Input: part model. Units: mm. Frame: model coordinates. A direction names the side the tool comes from. Round coordinates to 2 decimals unless told otherwise and drop trailing zeros. Order: outer loops, then holes, each group sorted by start corner. A loop starts at its lowest first (then second) coordinate and runs counter-clockwise, first axis right, second up. Notation, with made-up numbers: (-30.75, -11.5) -> (13.25, -11.5) arc R16 ccw to (13.25, 5.5) -> close; hole circle Ø6 at (89.5, 74.5). An arc over 180 degrees is marked (long way). Use a Markdown table: item, result.
Autodesk Inventor part; units mm, degrees
ref_plane "YZ Plane" through (0, 0, 0) normal (1, 0, 0) x (0, 1, 0)
ref_plane "XZ Plane" through (0, 0, 0) normal (0, 1, 0) x (-1, 0, 0)
ref_plane "XY Plane" through (0, 0, 0) normal (0, 0, 1) x (1, 0, 0)
sketch "Sketch1" plane through (0, 0, 0) normal (0, 1, 0) x (-1, 0, 0)
  circle A0 centre (0, 0) radius 1.5
  circle A1 centre (0, 0) radius 5.5
  circle A2 centre (0, -18) radius 5
  line L0 (5.4979, -0.1528) -> (4.9981, -18.1389)
  line L1 (-4.9981, -18.1389) -> (-5.4979, -0.1528)
  line L2 (0, 0) -> (0, 15) construction
  line L3 (-3.4, 0) -> (-3.4, 15)
  line L4 (3.4, 15) -> (3.4, 0)
  arc A3 (-3.4, 0) -> (3.4, 0) centre (0, 0) ccw
  arc A4 (3.4, 15) -> (-3.4, 15) centre (0, 15) ccw
  arc A5 (3.4, 7.5) -> (4.7003, 2.8561) centre (12.3429, 7.5) ccw
  arc A6 (-4.7003, 2.8561) -> (-3.4, 7.5) centre (-12.3429, 7.5) ccw
  point P0 (0, 7.5)
  point P1 (-3.4, 4.3232)
  point P2 (3.4, 4.3232)
  point P3 (-3.4, 7.5)
  dimension "d0" = 3
  dimension "d1" = 11
  dimension "d3" = 18
  dimension "d43" = 15
  dimension "d44" = 3.4
  dimension "d74" = 10
extrude "Extrusion1" add sketch "Sketch1" along normal blind 4
sketch "Sketch2" plane through (0, 4, 0) normal (0, 1, 0) x (1, 0, 0)
  arc A0 (4.9981, 18.1389) -> (-4.9981, 18.1389) centre (0, 18) ccw
  circle A1 centre (0, 0) radius 1.5
  line L0 (0, 16.8) -> (0, 12) construction
  line L1 (-2.6, 16.8) -> (-2.6, 12)
  line L2 (2.6, 12) -> (2.6, 16.8)
  arc A2 (2.6, 16.8) -> (-2.6, 16.8) centre (0, 16.8) ccw
  arc A3 (-2.6, 12) -> (2.6, 12) centre (0, 12) ccw
  line L3 (-3.4, -7.5) -> (-3.4, -15)
  arc A4 (-3.4, -15) -> (3.4, -15) centre (0, -15) ccw
  line L4 (3.4, -15) -> (3.4, -7.5)
  line L5 (-4.9981, 18.1389) -> (-5.4979, 0.1528)
  arc A5 (-5.4979, 0.1528) -> (-4.7003, -2.8561) centre (0, 0) ccw
  arc A6 (4.7003, -2.8561) -> (5.4979, 0.1528) centre (0, 0) ccw
  line L6 (5.4979, 0.1528) -> (4.9981, 18.1389)
  arc A7 (-3.4, -7.5) -> (-4.7003, -2.8561) centre (-12.3429, -7.5) ccw
  arc A8 (4.7003, -2.8561) -> (3.4, -7.5) centre (12.3429, -7.5) ccw
  point P0 (0, 14.4)
  dimension "d6" = 4.8
  dimension "d7" = 5.2
  dimension "d9" = 12
extrude "Extrusion2" cut sketch "Sketch2" against normal through all contours A2 L2 A3 L1
sketch "Sketch8" plane through (0, 4, 0) normal (0, 1, 0) x (1, 0, 0)
  line L0 (0, 31.28) -> (0, -26.68)
  line L1 (0, -14.5) -> (0, -7) construction
  line L2 (2.6, -14.5) -> (2.6, -7)
  line L3 (-2.6, -7) -> (-2.6, -14.5)
  arc A0 (-2.6, -14.5) -> (2.6, -14.5) centre (0, -14.5) ccw
  arc A1 (2.6, -7) -> (-2.6, -7) centre (0, -7) ccw
  point P0 (0, 0)
  point P1 (0, -10.75)
  dimension "d45" = 5.2
  dimension "d47" = 7
  dimension "d48" = 14.5
extrude "Extrusion8" cut sketch "Sketch8" against normal blind 1
sketch "Sketch10" plane through (0, 0, 0) normal (0, -1, 0) x (1, 0, 0)
  line L0 (0, 6.8) -> (0, 8.2) construction
  line L1 (1.1, 6.8) -> (1.1, 8.2)
  line L2 (-1.1, 8.2) -> (-1.1, 6.8)
  arc A0 (-1.1, 6.8) -> (1.1, 6.8) centre (0, 6.8) ccw
  arc A1 (1.1, 8.2) -> (-1.1, 8.2) centre (0, 8.2) ccw
  line L3 (0, 13) -> (0, 14.5) construction
  line L4 (1.1, 13) -> (1.1, 14.5)
  line L5 (-1.1, 14.5) -> (-1.1, 13)
  arc A2 (-1.1, 13) -> (1.1, 13) centre (0, 13) ccw
  arc A3 (1.1, 14.5) -> (-1.1, 14.5) centre (0, 14.5) ccw
  line L6 (0, -7.3) -> (0, -7.7) construction
  line L7 (1.1, -7.3) -> (1.1, -7.7)
  line L8 (-1.1, -7.7) -> (-1.1, -7.3)
  arc A4 (1.1, -7.3) -> (-1.1, -7.3) centre (0, -7.3) ccw
  arc A5 (-1.1, -7.7) -> (1.1, -7.7) centre (0, -7.7) ccw
  point P0 (0, 0)
  point P1 (0, 7.5)
  point P2 (0, 13.75)
  point P3 (0, -7.5)
  dimension "d60" = 2.2
  dimension "d61" = 6.8
  dimension "d62" = 1.4
  dimension "d63" = 1.5
  dimension "d64" = 2.2
  dimension "d65" = 13
  dimension "d78" = 0.2
  dimension "d79" = 7.5
extrude "Extrusion9" cut sketch "Sketch10" against normal through all contours A0 L2 A1 L1 | A2 L5 A3 L4
sketch "Sketch11" plane through (0, 0, 0) normal (0, -1, 0) x (1, 0, 0)
  circle A0 centre (0, 0) radius 4.25
  dimension "d73" = 8.5
extrude "Extrusion10" cut sketch "Sketch11" against normal blind 0.4
sketch "Sketch12" plane through (0, 4, 0) normal (0, 1, 0) x (1, 0, 0)
  circle A0 centre (0, 0) radius 2.5
  dimension "d75" = 5
extrude "Extrusion11" cut sketch "Sketch12" against normal blind 1
properties part number "Servo steering actuator v2"
1) Cut plane D-D on z = 16. Return loops of the section in (x, y).
Answer key:
| item | result |
|---|---|
| outline | (-3.25, 0) -> (3.25, 0) -> (3.25, 4) -> (2.12, 4) -> (2.12, 3) -> (-2.12, 3) -> (-2.12, 4) -> (-3.25, 4) -> close |
2) Set-up query: faces 3 (the face through (2, 3, 0)), 4 (the face through (1.1, 1, 7)), 5 (the face through (2.285, 0.197, 3.584)). Return all of +Z, -Z, +X, -X, +Y, -Y with unobstructed straight access to the full face (end or side cutting, diameter ignored); none if empty.
Answer key:
| item | result |
|---|---|
| face 3 | +Y |
| face 4 | +Y, -Y |
| face 5 | -Y |
3) Ray query, probe 1 along Z at (x, y) = (0, 2.45); probe 2 along Z at (x, y) = (0, 3.7); probe 3 along X at (y, z) = (2.7, 13). Return the intervals inside material, ascending.
Answer key:
| item | result |
|---|---|
| probe 1 | z = -23 to -19.4, -9.4 to -1.5, 1.5 to 5.7, 9.3 to 11.9, 15.6 to 18.4 |
| probe 2 | z = -23 to -19.4, -9.4 to -2.5, 2.5 to 4.4, 17.1 to 18.4 |
| probe 3 | x = -3.4 to -1.1, 1.1 to 3.4 |
4) Contact query for flat-ended pins moving along their axis: P1, Ø1.6, axis at y = 1, z = 13.5, coming from the -X side; P2, Ø4, axis at x = 0, z = 8, coming from the +Y side; P3, Ø2, axis at y = 2, z = 8.5, coming from the +X side. Output: stop coordinate, or through.
Answer key:
| item | result |
|---|---|
| P1 | stops at x = -3.4 |
| P2 | stops at y = 3 |
| P3 | stops at x = 3.4 |
5) Cut plane C-C on y = 1.5. Return loops of the section in (x, z), and give its area (3 significant figures).
Answer key:
| item | result |
|---|---|
| outline | (-5.5, -0.15) -> (-5, -18) arc R5 ccw to (5, -18.14) -> (5.5, -0.15) arc R5.5 ccw to (4.7, 2.86) arc R8.94 cw to (3.4, 7.5) -> (3.4, 15) arc R3.4 ccw to (-3.4, 15) -> (-3.4, 7.5) arc R8.94 cw to (-4.7, 2.86) arc R5.5 ccw to start; hole (-2.6, -16.8) arc R2.6 ccw to (2.6, -16.8) -> (2.6, -12) arc R2.6 ccw to (-2.6, -12) -> close; hole circle Ø3 at (0, 0); hole (-1.1, 6.8) arc R1.1 ccw to (1.1, 6.8) -> (1.1, 8.2) arc R1.1 ccw to (-1.1, 8.2) -> close; hole (-1.1, 13) arc R1.1 ccw to (1.1, 13) -> (1.1, 14.5) arc R1.1 ccw to (-1.1, 14.5) -> close |
| area | 296 mm^2 |
6) Cut plane B-B on z = -11. Return loops of the section in (x, y).
Answer key:
| item | result |
|---|---|
| outline | (-5.2, 0) -> (-2.4, 0) -> (-2.4, 4) -> (-5.2, 4) -> close; (2.4, 0) -> (5.2, 0) -> (5.2, 4) -> (2.4, 4) -> close |
7) Draft query along X for faces 1 (the face through (-2.6, 3.5, 10.7)), 2 (the face through (-3.4, 2, 11)). Return one class per face: released by +X, released by -X, zero draft, split by the parting line, or undercut.
Answer key:
| item | result |
|---|---|
| face 1 | undercut |
| face 2 | released by -X |
8) Cut plane A-A on x = 0. State how many separate pieces and enclosed holes the cut face has, and give its area (3 significant figures).
Answer key:
| item | result |
|---|---|
| separate pieces | 5 |
| enclosed holes | 0 |
| area | 74.8 mm^2 |
